Can you work these out from the drawing? Everything is in mm from the part's minimum corner. A direction names the side the tool comes from. Coordinates: 2 decimals unless noted, no trailing zeros. Order: outer loops, then holes, each group sorted by start corner. A loop starts at its lowest first (then second) coordinate and runs counter-clockwise, first axis right, second up. Notation, with made-up numbers: (88, -5.5) -> (105, -5.5) arc R21 ccw to (105, 18.5) -> close; hole circle Ø10 at (73, 6). An arc over 180 degrees is marked (long way). Return JSON: item names as keys, results as strings. Group by question number.
1) If we section it at B-B, the plane z = 5.5: Please give me the cut outline in (x, y), then the cut area to 3 significant figures.
2) If we section it at A-A, the plane x = 30.5: Please give me the cut outline in (y, z), then the cut area to 3 significant figures.
3) If I drill on probe 1 along X at (y, z) = (3.25, 6.5); probe 2 along X at (y, z) = (4, 8); probe 3 along Y at (x, z) = (30.5, 3.5), over which ranges is the centre line in solid material (lowest first)? Write a range as from..to.
4) For pin 1 (5.5 mm diameter, centred on x = 21.5, z = 4.5, fed in from -Y); pin 2 (1.3 mm diameter, centred on x = 35, z = 8, fed in from +Y); pin 3 (0.8 mm diameter, centred on x = 35, z = 7.5, fed in from -Y), each with a flat end and sliding along its axis, tell me the tip position at first contact or that it passes through.
5) If we section it at C-C, the plane y = 8.25: Please give me the cut outline in (x, z), then the cut area to 3 significant figures.
6) For the marked faces 1 and 2, which set-ups out of +Z, -Z, +X, -X, +Y, -Y let a thin tool reach every point of the face, with its end or its side?
7) Thinking about a two-plate mould opening in X: for the marked faces 3 and 4, which applies, +X half, -X half, draft (parallel to the pull), parting line (faces both ways), or undercut?
8) If we section it at D-D, the plane x = 12: Please give me the cut outline in (y, z), then the cut area to 3 significant figures.
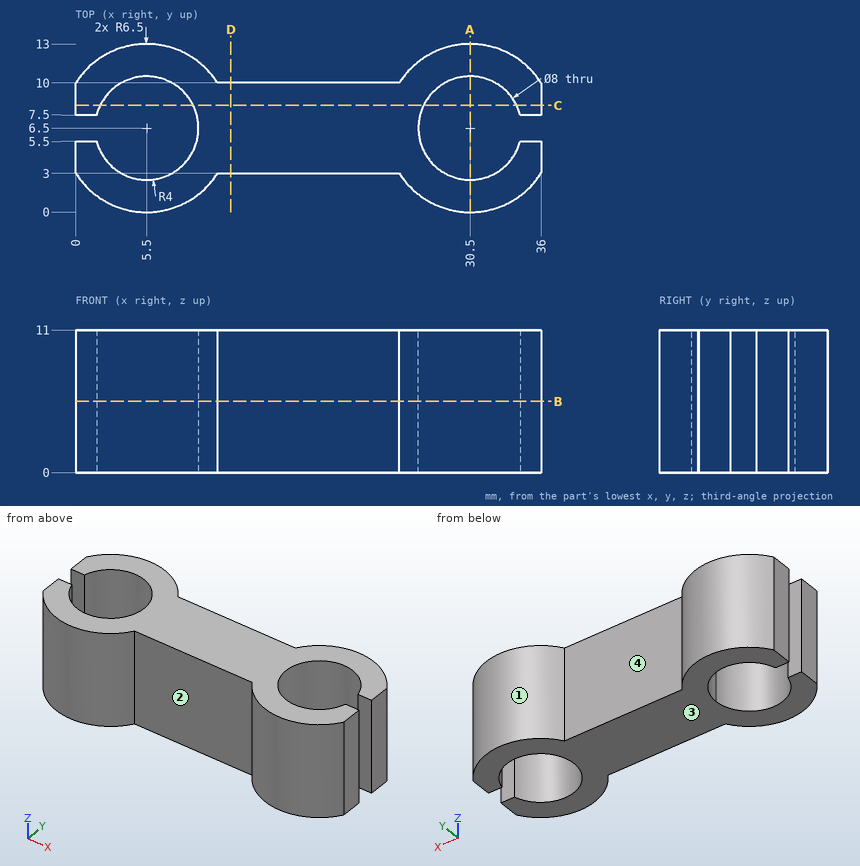
Result sheet:
{
 "1": {"outline": "(0, 3.04) arc R6.5 ccw to (10.98, 3) -> (25.02, 3) arc R6.5 ccw to (36, 3.04) -> (36, 5.5) -> (34.37, 5.5) arc R4 cw (long way) to (34.37, 7.5) -> (36, 7.5) -> (36, 9.96) arc R6.5 ccw to (25.02, 10) -> (10.98, 10) arc R6.5 ccw to (0, 9.96) -> (0, 7.5) -> (1.63, 7.5) arc R4 cw (long way) to (1.63, 5.5) -> (0, 5.5) -> close", "area": "238 mm2"},
 "2": {"outline": "(0, 0) -> (2.5, 0) -> (2.5, 11) -> (0, 11) -> close; (10.5, 0) -> (13, 0) -> (13, 11) -> (10.5, 11) -> close", "area": "55.0 mm2"},
 "3": {"probe 1": "x = 0..3.17, 7.83..28.17, 32.83..36", "probe 2": "x = 0..2.38, 8.62..27.38, 33.62..36", "probe 3": "y = 0..2.5, 10.5..13"},
 "4": {"pin 1": "stops at y = 3", "pin 2": "stops at y = 11.74", "pin 3": "stops at y = 1.46"},
 "5": {"outline": "(0, 0) -> (1.9, 0) -> (1.9, 11) -> (0, 11) -> close; (9.1, 0) -> (26.9, 0) -> (26.9, 11) -> (9.1, 11) -> close; (34.1, 0) -> (36, 0) -> (36, 11) -> (34.1, 11) -> close", "area": "238 mm2"},
 "6": {"face 1": "+Z, -Z, +Y", "face 2": "+Z, -Z, -Y"},
 "7": {"face 3": "draft", "face 4": "undercut"},
 "8": {"outline": "(3, 0) -> (10, 0) -> (10, 11) -> (3, 11) -> close", "area": "77.0 mm2"}
}
